Check sheet for the drawn part. Datum: minimum x, y, z corner. Units: mm. A direction names the side the tool comes from. Coordinates: 2 decimals unless noted, no trailing zeros. Write each loop counter-clockwise with the first axis right and the second up, starting at its lowest first coordinate (ties: lowest second). Pieces come first, ordered by that corner, then holes. Notation, with made-up numbers: (29.25, 6) -> (87.25, 6) arc R19 cw to (87.25, 35) -> close; hole circle Ø8 at (83, 62.5). An arc over 180 degrees is marked (long way). One line per question, with ' | ' between items.
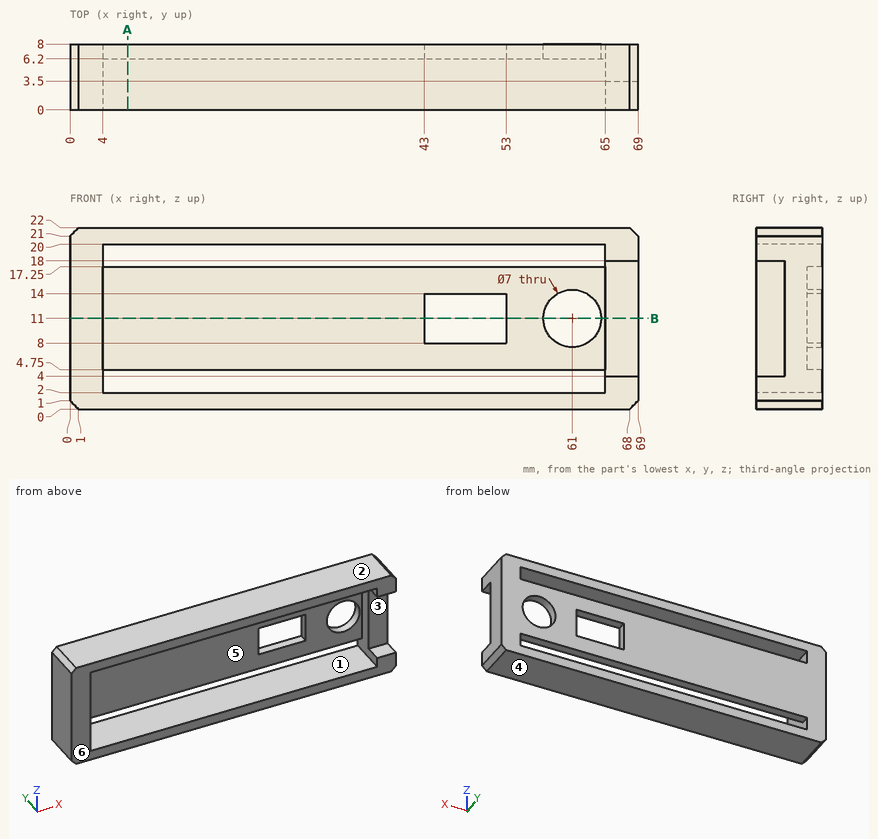
1. Material ranges on line 1 (X direction, y = 7.45, z = 11); line 2 (Z direction, x = 14, y = 6.5); line 3 (Z direction, x = 22, y = 0.75), recorded low to high. Write a range as from..to.
Worked answers:
line 1: 0..43, 53..57.5, 64.5..69 | line 2: 0..2, 4.75..17.25, 20..22 | line 3: 0..2, 20..22
2. Cross-section at A-A on x = 7. Record the boundary of the cut face in (y, z), and give its area (3 significant figures).
Worked answers:
outline: (0, 0) -> (8, 0) -> (8, 2) -> (0, 2) -> close; (0, 20) -> (8, 20) -> (8, 22) -> (0, 22) -> close; (6.2, 4.75) -> (8, 4.75) -> (8, 17.25) -> (6.2, 17.25) -> close | area: 54.5 mm²
3. Mould release check, pull along Z, two halves, no side actions. Record for the marked faces 4, 5 and 6: released by +Z, released by -Z, zero draft, split by the parting line, or undercut.
Worked answers:
face 4: released by -Z | face 5: undercut | face 6: zero draft
4. Cross-section at B-B on z = 11. Record the boundary of the cut face in (x, y), and give its area (3 significant figures).
Worked answers:
outline: (0, 0) -> (4, 0) -> (4, 6.2) -> (43, 6.2) -> (43, 8) -> (0, 8) -> close; (53, 6.2) -> (57.5, 6.2) -> (57.5, 8) -> (53, 8) -> close; (64.5, 6.2) -> (65, 6.2) -> (65, 3.5) -> (69, 3.5) -> (69, 8) -> (64.5, 8) -> close | area: 129 mm²
5. Go/stop test with flat-tipped pins: P1, Ø2, axis at y = 7.5, z = 10, coming from the -X side; P2, Ø1.5, axis at x = 18, z = 12.5, coming from the -Y side; P3, Ø2, axis at y = 1, z = 10, coming from the +X side; P4, Ø2, axis at x = 66.5, z = 8, coming from the -Y side. Record where each tip stops, or that it passes through.
Worked answers:
P1: x = 0 | P2: y = 6.2 | P3: x = 4 | P4: y = 3.5
6. Tool access check on the marked faces 1, 2 and 3. Record the directions out of +Z, -Z, +X, -X, +Y, -Y that give a thin tool (end or side, any length) a straight path to the whole face; none if there is none.
Worked answers:
face 1: +Y, -Y | face 2: +Z, +X, -X, +Y, -Y | face 3: +X, -Y
